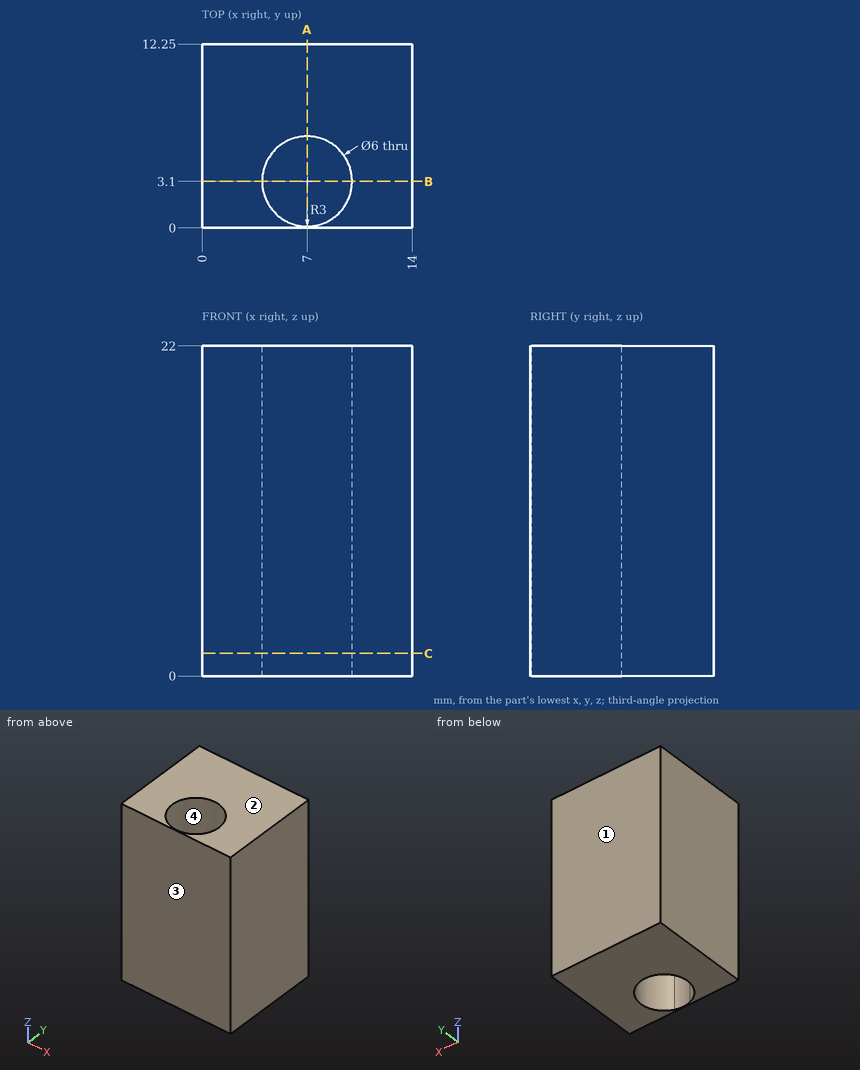
Job drawing, mm, ordinate dimensions from the low corner. One solid piece. Round coordinates to 2 decimals unless told otherwise and drop trailing zeros. Write each loop counter-clockwise with the first axis right and the second up, starting at its lowest first coordinate (ties: lowest second). Pieces come first, ordered by that corner, then holes. Notation, with made-up numbers: (-22, -19) -> (-12, -19) arc R28 cw to (-12, 6) -> close; hole circle Ø1 at (50.5, 16.25). An arc over 180 degrees is marked (long way). Answer as a JSON object with one key per item and string values.
(1) Two-plate mould, pull along Y, no slides. Class the marked faces 1, 2, 3 and 4: +Y half, -Y half, draft (parallel to the pull), parting line (faces both ways), or undercut.
Reported:
{"face 1": "+Y half", "face 2": "draft", "face 3": "-Y half", "face 4": "undercut"}
(2) Band-saw the part on A-A, the plane x = 7. List the corners of the cut face in (y, z).
Reported:
{"outline": "(0, 0) -> (0.1, 0) -> (0.1, 22) -> (0, 22) -> close; (6.1, 0) -> (12.25, 0) -> (12.25, 22) -> (6.1, 22) -> close"}
(3) Pin check, flat tip, straight feed: P1, Ø1.5, axis at y = 10, z = 11, coming from the -X side. Stop position of the tip, or through.
Reported:
{"P1": "stops at x = 0"}
(4) Probe probe 1 along X at (y, z) = (3.1, 17); probe 2 along X at (y, z) = (5.25, 18.5); probe 3 along Y at (x, z) = (5.5, 19.5). List the from-to ranges inside material, lowest first. Write a range as [from, to].
Reported:
{"probe 1": "x = [0, 4], [10, 14]", "probe 2": "x = [0, 4.91], [9.09, 14]", "probe 3": "y = [0, 0.5], [5.7, 12.25]"}
(5) Band-saw the part on B-B, the plane y = 3.1. List the corners of the cut face in (x, z), then the cut area to 3 significant figures.
Reported:
{"outline": "(0, 0) -> (4, 0) -> (4, 22) -> (0, 22) -> close; (10, 0) -> (14, 0) -> (14, 22) -> (10, 22) -> close", "area": "176 mm^2"}
(6) Band-saw the part on C-C, the plane z = 1.5. List the corners of the cut face in (x, y).
Reported:
{"outline": "(0, 0) -> (14, 0) -> (14, 12.25) -> (0, 12.25) -> close; hole circle Ø6 at (7, 3.1)"}
